Autodesk Inventor part; units mm, degrees
ref_plane "YZ Plane" through (0, 0, 0) normal (1, 0, 0) x (0, 1, 0)
ref_plane "XZ Plane" through (0, 0, 0) normal (0, 1, 0) x (-1, 0, 0)
ref_plane "XY Plane" through (0, 0, 0) normal (0, 0, 1) x (1, 0, 0)
sketch "Sketch1" plane through (0, 0, 0) normal (0, 1, 0) x (-1, 0, 0)
  line L0 (-60, 60) -> (60, 60)
  line L1 (60, 60) -> (60, -60)
  line L2 (60, -60) -> (-60, -60)
  line L3 (-60, -60) -> (-60, 60)
  line L4 (-60, 60) -> (60, -60) construction
  line L5 (60, 60) -> (-60, -60) construction
  point P0 (0, 0)
  dimension "d2" = 120
  dimension "d3" = 120
extrude "Extrusion1" add sketch "Sketch1" along normal blind 10
sketch "Sketch2" plane through (0, 10, 0) normal (0, 1, 0) x (1, 0, 0)
  line L0 (-50, -43) -> (6, -43)
  line L1 (6, -43) -> (6, 43)
  line L2 (6, 43) -> (-50, 43)
  line L3 (-50, 43) -> (-50, -43)
  line L4 (-60, 60) -> (-60, -60)
  line L5 (-60, -60) -> (60, -60)
  line L6 (16, -52.5) -> (48, -52.5)
  line L7 (48, -52.5) -> (48, 9.45)
  line L8 (48, 9.45) -> (16, 9.45)
  line L9 (16, 9.45) -> (16, -52.5)
  line L10 (23.25, 21.45) -> (40.75, 21.45)
  line L11 (40.75, 21.45) -> (40.75, 44.95)
  line L12 (40.75, 44.95) -> (23.25, 44.95)
  line L13 (23.25, 44.95) -> (23.25, 21.45)
  line L14 (8.5, -43) -> (15, -43)
  line L15 (15, -43) -> (15, -31)
  line L16 (15, -31) -> (8.5, -31)
  line L17 (8.5, -31) -> (8.5, -43)
  line L18 (8.5, 43) -> (15, 43)
  line L19 (15, 43) -> (15, 31)
  line L20 (15, 31) -> (8.5, 31)
  line L21 (8.5, 31) -> (8.5, 43)
  point P0 (0, 0)
  point P1 (32, 21.45)
  point P2 (32, 9.45)
  point P3 (-50, 0)
  point P4 (-60, 0)
  dimension "d4" = 86
  dimension "d5" = 56
  dimension "d6" = 10
  dimension "d8" = 61.95
  dimension "d9" = 32
  dimension "d10" = 10
  dimension "d11" = 7.5
  dimension "d12" = 23.5
  dimension "d13" = 17.5
  dimension "d14" = 12
  dimension "d40" = 6.5
  dimension "d41" = 12
  dimension "d42" = 6.5
  dimension "d43" = 12
  dimension "d44" = 1
fillet "Fillet1" radius 5 4 edges at (60, 5, -60) (60, 5, 60) (-60, 5, -60) (-60, 5, 60)
sketch "Sketch3" plane through (0, 0, 0) normal (0, -1, 0) x (1, 0, 0)
  circle A0 centre (21.5, 25.35) radius 2.675
  circle A1 centre (41.5, 25.35) radius 2.675
  circle A2 centre (28.25, -38.7) radius 2.675
  circle A3 centre (35.75, -26.45) radius 2.675
  circle A4 centre (43, -4.45) radius 2.675
  circle A5 centre (20, -4.45) radius 2.675
  circle A6 centre (53, 33) radius 2.675
  circle A7 centre (53, -33) radius 2.675
  circle A8 centre (-53, 53) radius 2.675
  circle A9 centre (-53, -53) radius 2.675
  circle A10 centre (11.75, 37) radius 2.675
  circle A11 centre (11.75, -37) radius 2.675
  point P0 (0, 0)
hole "Hole1" at (41.5, 0, 25.35) at (43, 0, -4.45) at (35.75, 0, -26.45) at (28.25, 0, -38.7) at (20, 0, -4.45) at (21.5, 0, 25.35) at (53, 0, 33) at (-53, 0, 53) at (-53, 0, -53) at (53, 0, -33) at (11.75, 0, 37) at (11.75, 0, -37) direction (0, 1, 0) diameter 4.7 end through all counterbore diameter 9 counterbore depth 4
sketch "Sketch4" plane through (55, 0, -60) normal (0, 0, -1) x (-1, 0, 0)
  line L0 (-5, 10) -> (-5, 0)
  line L1 (-5, 7.5) -> (95, 7.5)
  line L2 (95, 7.5) -> (95, 2.5)
  line L3 (95, 2.5) -> (-5, 2.5)
  line L4 (-5, 2.5) -> (-5, 7.5)
  point P0 (55, 0)
  point P1 (-5, 5)
  point P2 (-5, 5)
  point P3 (-5, 2.5)
  dimension "d23" = 5
  dimension "d24" = 100
extrude "Extrusion2" cut sketch "Sketch4" against normal blind 10
sketch "Sketch5" plane through (-40, 7.5, -60) normal (0, -1, 0) x (1, 0, 0)
  arc A0 (17.5, 3) -> (12.5, 3) centre (15, 3) ccw
  line L0 (17.5, 3) -> (17.5, 0)
  line L1 (12.5, 3) -> (12.5, 0)
  line L2 (14, 0) -> (14, 3)
  arc A1 (16, 3) -> (14, 3) centre (15, 3) ccw
  line L3 (16, 3) -> (16, 0)
  line L4 (17.5, 0) -> (16, 0)
  line L5 (95, 0) -> (0, 0)
  line L6 (14, 0) -> (12.5, 0)
  line L7 (100, 10) -> (100, 5)
  point P0 (40, 60)
  dimension "d27" = 5
  dimension "d31" = 1.5
  dimension "d34" = 3
  dimension "d35" = 85
  dimension "d36" = 5
extrude "Extrusion3" add sketch "Sketch5" along normal blind 2 contours L0 L4 L3 A1 L2 L5 L1 A0
pattern_linear "Rectangular Pattern1" count 2 spacing 60 along (1, 0, 0) of "Extrusion3"
ref_plane "Work Plane1" through (55, 0, 0) normal (0, 0, -1) x (-1, 0, 0)
mirror "Mirror1" about plane through (55, 0, 0) normal (0, 0, -1) of "Extrusion2", "Extrusion3", "Rectangular Pattern1"
properties part number "PCB_Housing_01_003"
Geometry check sheet. Reference: the model listing, model coordinates, mm. A direction names the side the tool comes from. Round coordinates to 2 decimals unless told otherwise and drop trailing zeros. Write each loop counter-clockwise with the first axis right and the second up, starting at its lowest first coordinate (ties: lowest second). Pieces come first, ordered by that corner, then holes. Notation, with made-up numbers: (-7, -26.75) - (42, -26.75) arc R23 cw to (42, 3.25) - close; hole circle Ø8 at (-15.75, -6). An arc over 180 degrees is marked (long way). One line per item, written item: value.
1. Depth check by flat-ended pin: pin 1 Ø10 at (x, z) = (12, -37.5) entering from -Y; pin 2 Ø2.5 at (x, y) = (30, 5.5) entering from +Z; pin 3 Ø2.5 at (x, z) = (52.5, 31.5) entering from -Y; pin 4 Ø0.6 at (y, z) = (6.5, 58.5) entering from -X. Enter the tip coordinate at first touch or a pass-through.
The answers:
pin 1: stops at y = 0
pin 2: stops at z = 50
pin 3: stops at y = 4
pin 4: stops at x = -58.84
2. Set-up check for faces 4 (the face through (-40, 5, -55)), 5 (the face through (45.9, 2, 26.3)), 6 (the face through (23.585, 7.042, 24.266)), 7 (the face through (1, 10, 1)), 8 (the face through (-23.9, 5.5, -56.6)): record each of +Z, -Z, +X, -X, +Y, -Y from which the full face is reachable in a straight line by a thin tool's end or side.
The answers:
face 4: -Z
face 5: -Y
face 6: +Y, -Y
face 7: +Z, -Z, +X, -X, +Y
face 8: -Z, +X
3. Mould release check, pull along Z, two halves, no side actions. Record for faces 1 (the face through (59, 1, -58)), 2 (the face through (39.518, 7.042, 24.087)), 3 (the face through (33.9, 5.5, 56.6)): released by +Z, released by -Z, zero draft, split by the parting line, or undercut.
The answers:
face 1: released by -Z
face 2: undercut
face 3: zero draft
4. Cross-section at A-A on z = -26.45. Record the boundary of the cut face in (x, y), and give its area (3 significant figures).
The answers:
outline: (-60, 0) - (31.25, 0) - (31.25, 4) - (33.4, 4) - (33.4, 10) - (-60, 10) - close; (38.1, 4) - (40.25, 4) - (40.25, 0) - (60, 0) - (60, 10) - (38.1, 10) - close
area: 1,140 mm^2
5. Scan lines: L1, parallel to Z at x = 53, y = 6.1; L2, parallel to Y at x = 1, z = -54.5; L3, parallel to X at y = 2.55, z = -4.45. Record each from-to range of solid material in increasing order.
The answers:
L1: z = -50 to -35.35, -30.65 to 30.65, 35.35 to 50
L2: y = 0 to 2.5, 7.5 to 10
L3: x = -60 to 15.5, 24.5 to 38.5, 47.5 to 60
6. Cross-section at C-C on z = -4.45. Record the boundary of the cut face in (x, y).
The answers:
outline: (-60, 0) - (15.5, 0) - (15.5, 4) - (17.65, 4) - (17.65, 10) - (-60, 10) - close; (22.35, 4) - (24.5, 4) - (24.5, 0) - (38.5, 0) - (38.5, 4) - (40.65, 4) - (40.65, 10) - (22.35, 10) - close; (45.35, 4) - (47.5, 4) - (47.5, 0) - (60, 0) - (60, 10) - (45.35, 10) - close
7. Cross-section at B-B on x = 28.25. Record the boundary of the cut face in (y, z).
The answers:
outline: (0, -60) - (2.5, -60) - (2.5, -50) - (7.5, -50) - (7.5, -60) - (10, -60) - (10, -41.05) - (4, -41.05) - (4, -43.2) - (0, -43.2) - close; (0, -34.2) - (4, -34.2) - (4, -36.35) - (10, -36.35) - (10, 60) - (7.5, 60) - (7.5, 50) - (2.5, 50) - (2.5, 60) - (0, 60) - close
8. Cross-section at D-D on x = 11.75. Record the boundary of the cut face in (y, z), and give its area (3 significant figures).
The answers:
outline: (0, -60) - (2.5, -60) - (2.5, -50) - (7.5, -50) - (7.5, -60) - (10, -60) - (10, -39.35) - (4, -39.35) - (4, -41.5) - (0, -41.5) - close; (0, -32.5) - (4, -32.5) - (4, -34.65) - (10, -34.65) - (10, 34.65) - (4, 34.65) - (4, 32.5) - (0, 32.5) - close; (0, 41.5) - (4, 41.5) - (4, 39.35) - (10, 39.35) - (10, 60) - (7.5, 60) - (7.5, 50) - (2.5, 50) - (2.5, 60) - (0, 60) - close
area: 972 mm^2
